from build123d import *

# Parameters (mm, degrees)
F2_T     = -1
F3_R     = 113
F4_DEPTH = 200.001
F5_W     = 200
F5_H     = 140
F6_DEPTH = 100.001


with BuildPart() as f1:
    # F0 (on Front) → F1 (revolve)
    with BuildSketch(Plane.XZ):
        Polygon((0, 100), (-115, 100), (-115, 0), (-330, 0), (-330, -100), (0, -100), align=None)
    revolve(axis=Axis((0, 0, 94.9130495359), (0, 0, 1)))

    # F2
    f2_openings = [f1.faces().sort_by_distance(p)[0] for p in [
        (0, 0, -100),
    ]]
    offset(amount=F2_T, openings=f2_openings, kind=Kind.INTERSECTION)

    # F3 (on face) → F4 (cut, through all)
    with BuildSketch(Plane.XY.offset(100)):
        Circle(F3_R)
    extrude(amount=-F4_DEPTH, mode=Mode.SUBTRACT)

    # F5 (on face) → F6 (cut, through all)
    with BuildSketch(Plane.XY):
        with Locations((0, -210)):
            Rectangle(F5_W, F5_H)
    extrude(amount=-F6_DEPTH, mode=Mode.SUBTRACT)


solid = f1.part
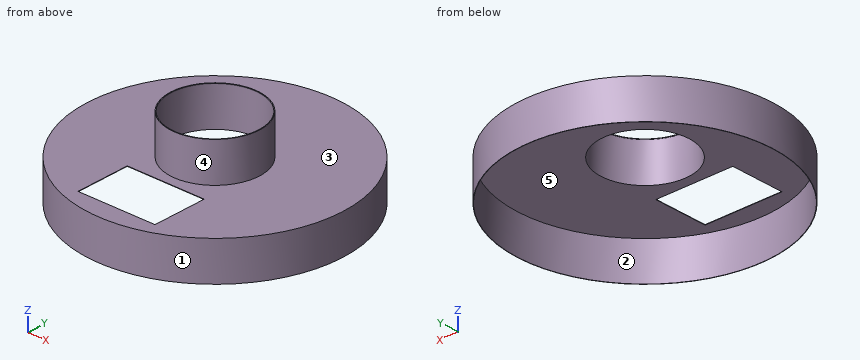
Could you check a few things on this model? Use its own coordinates, in mm. Face numbers are marked on the shaded views. A direction names the side the tool comes from. Round coordinates to 2 decimals unless told otherwise and drop trailing zeros. Loops run counter-clockwise (first coordinate to the right, second up) from the corner with the lowest first, then second, coordinate; pieces in that order, holes last. Notation, with made-up numbers: (57.25, 77.25) -> (111.25, 77.25) arc R27 cw to (111.25, 97.25) -> close; hole circle Ø9 at (31.5, 25). An arc over 180 degrees is marked (long way). Use CSV: the item, a comma, the result in double quotes.
(1) For the marked faces 1 and 2, which set-ups out of +Z, -Z, +X, -X, +Y, -Y let a thin tool reach every point of the face, with its end or its side?
Return value:
face 1,"+Z, -Z"
face 2,"-Z"
(2) Suppose I cut it at B-B on y = 0. Write out the boundary of the cut face in (x, z).
Return value:
outline,"(-330, -100) -> (-329, -100) -> (-329, -1) -> (-114, -1) -> (-114, 99) -> (-113, 99) -> (-113, 100) -> (-115, 100) -> (-115, 0) -> (-330, 0) -> close; (113, 99) -> (114, 99) -> (114, -1) -> (329, -1) -> (329, -100) -> (330, -100) -> (330, 0) -> (115, 0) -> (115, 100) -> (113, 100) -> close"
(3) If we mould it in two halves opening along X, with no side actions, what happens to the marked faces 3, 4 and 5? For each: +X half, -X half, draft (parallel to the pull), parting line (faces both ways), or undercut.
Return value:
face 3,"draft"
face 4,"parting line"
face 5,"undercut"
(4) If I drill on probe 1 along Y at (x, z) = (0, -78); probe 2 along Y at (x, z) = (0, 43); probe 3 along Z at (x, y) = (-279.5, -18), over which ranges is the centre line in solid material (lowest first)? Write a range as [from, to].
Return value:
probe 1,"y = [-330, -329], [329, 330]"
probe 2,"y = [-115, -114], [114, 115]"
probe 3,"z = [-1, 0]"
(5) Suppose I cut it at A-A on x = 0. Write out the boundary of the cut face in (y, z).
Return value:
outline,"(-330, -100) -> (-329, -100) -> (-329, -1) -> (-280, -1) -> (-280, 0) -> (-330, 0) -> close; (-140, -1) -> (-114, -1) -> (-114, 99) -> (-113, 99) -> (-113, 100) -> (-115, 100) -> (-115, 0) -> (-140, 0) -> close; (113, 99) -> (114, 99) -> (114, -1) -> (329, -1) -> (329, -100) -> (330, -100) -> (330, 0) -> (115, 0) -> (115, 100) -> (113, 100) -> close"
(6) Suppose I cut it at D-D on y = 262.5. Write out the boundary of the cut face in (x, z).
Return value:
outline,"(-199.98, -100) -> (-198.33, -100) -> (-198.33, -1) -> (198.33, -1) -> (198.33, -100) -> (199.98, -100) -> (199.98, 0) -> (-199.98, 0) -> close"
(7) Suppose I cut it at C-C on z = -65. Write out the boundary of the cut face in (x, y).
Return value:
outline,"circle Ø660 at (0, 0); hole circle Ø658 at (0, 0)"
(8) Will these pins go through, and if not, where does the flat tip stop? pin 1 Ø8 at (x, y) = (-157, -207) entering from +Z; pin 2 Ø12 at (x, y) = (-47.5, 190.5) entering from -Z; pin 3 Ø5 at (y, z) = (83, -75.5) entering from +X.
Return value:
pin 1,"stops at z = 0"
pin 2,"stops at z = -1"
pin 3,"stops at x = 320.03"
